```python
from build123d import *

# Parameters (mm, degrees)
F1_DEPTH = 19.05
F3_DEPTH = 38.1


with BuildPart() as f1:
    # F0 (on Front) → F1 (new body)
    with BuildSketch(Plane.XZ):
        Polygon((25.603199, 0), (-75.996801, 0), (-75.996801, -63.5), (51.003199, -63.5), (51.003199, -25.4), align=None)
    extrude(amount=F1_DEPTH)

    # F2 (on Front) → F3 (join)
    with BuildSketch(Plane.XZ):
        Polygon((-50.5968, 0), (-76.200001, 0), (-76.200001, -63.246004), (12.8016, -63.246004), align=None)
    extrude(amount=F3_DEPTH)


solid = f1.part
```
Part model, mm, in its own coordinate system. A direction names the side the tool comes from. Round coordinates to 2 decimals unless told otherwise and drop trailing zeros. Write each loop counter-clockwise with the first axis right and the second up, starting at its lowest first coordinate (ties: lowest second). Pieces come first, ordered by that corner, then holes. Notation, with made-up numbers: M 65.25,83.5 L 101.25,83.5 A34 cw 101.25,120.5 Z; hole C 32,-12.5 d3. An arc over 180 degrees is marked long. One line per question, with ' | ' between items.
(1) Saw through at A-A on y = -10.5. Write the cut outline in (x, z), then the cut area to 3 significant figures.
Answer key:
outline: M -76.2,-63.25 L -76,-63.25 L -76,-63.5 L 51,-63.5 L 51,-25.4 L 25.6,0 L -76.2,0 Z | area: 7,750 mm^2
(2) 3-axis set-ups, long thin cutter, end or side, ignore diameter. For faces 1 (the face through (51.003, -9, -45)), 2 (the face through (-18.45, -28.44, -32.07)): which of +Z, -Z, +X, -X, +Y, -Y reach the whole face in a straight line?
Answer key:
face 1: +Z, -Z, +X, +Y, -Y | face 2: +Z, +X, -Y
(3) Pin check, flat tips, straight feed: pin 1 (5 mm diameter, centred on y = -22.5, z = -17.5, fed in from +X); pin 2 (10 mm diameter, centred on x = 36.5, z = -45, fed in from -Y); pin 3 (2 mm diameter, centred on y = -29.5, z = -32, fed in from +X). Stop position of each tip, or through.
Answer key:
pin 1: stops at x = -30.55 | pin 2: stops at y = -19.05 | pin 3: stops at x = -17.52
(4) Saw through at D-D on y = -23.5. Write the cut outline in (x, z), then the cut area to 3 significant figures.
Answer key:
outline: M -76.2,-63.25 L 12.8,-63.25 L -50.6,0 L -76.2,0 Z | area: 3,620 mm^2
(5) Saw through at B-B on x = -36. Write the cut outline in (y, z), then the cut area to 3 significant figures.
Answer key:
outline: M -38.1,-63.25 L -19.05,-63.25 L -19.05,-63.5 L 0,-63.5 L 0,0 L -19.05,0 L -19.05,-14.56 L -38.1,-14.56 Z | area: 2,140 mm^2
(6) Saw through at C-C on z = -7. Write the cut outline in (x, y).
Answer key:
outline: M -76.2,-38.1 L -43.58,-38.1 L -43.58,-19.05 L 32.6,-19.05 L 32.6,0 L -76.2,0 Z
(7) Probe line 1 along Y through (x, z) = (41, -29); line 2 along Z through (x, y) = (-54, -30.5); line 3 along X through (y, z) = (-19.5, -31.5). List the from-to ranges inside material, lowest first.
Answer key:
line 1: y = -19.05 to 0 | line 2: z = -63.25 to 0 | line 3: x = -76.2 to -19.02
